Geometry: see drawing. Coordinates: mm, zero at the bounding-box minimum. A direction names the side the tool comes from. Round coordinates to 2 decimals unless told otherwise and drop trailing zeros. Loops run counter-clockwise (first coordinate to the right, second up) from the corner with the lowest first, then second, coordinate; pieces in that order, holes last.
(1) Set-up query: the marked faces 5 and 6. Return all of +Z, -Z, +X, -X, +Y, -Y with unobstructed straight access to the full face (end or side cutting, diameter ignored); none if empty.
(2) Section C-C, the plane x = 42.5. Return the cut outline in (y, z), plus the area to 3 significant figures.
(3) Material intervals for probe 1 along Y at (x, z) = (7.5, 13) (1 decimal); probe 2 along Y at (x, z) = (22, 44); probe 3 along X at (y, z) = (31.5, 40.5), sorted ascending.
(4) Section A-A, the plane z = 50.5. Return the cut outline in (x, y).
(5) Mould query, pull axis Y, two halves, no side actions, for the marked faces 1, 2, 3 and 4. Classes: pulls with the +Y half, pulls with the -Y half, needs draft (parallel to the pull), parting line crosses it, or undercut.
(6) Section B-B, the plane y = 40. Return the cut outline in (x, z), plus the area to 3 significant figures.
(7) Section D-D, the plane z = 32. Return the cut outline in (x, y).
(8) First-contact query: pin 1 Ø12 at (y, z) = (16.5, 15.5) entering from +X; pin 2 Ø6 at (y, z) = (41, 7.5) entering from -X; pin 3 Ø1.5 at (x, z) = (45, 35.5) entering from +Y. Flat tips, straight axial feed; report the tip coordinate or a pass-through.
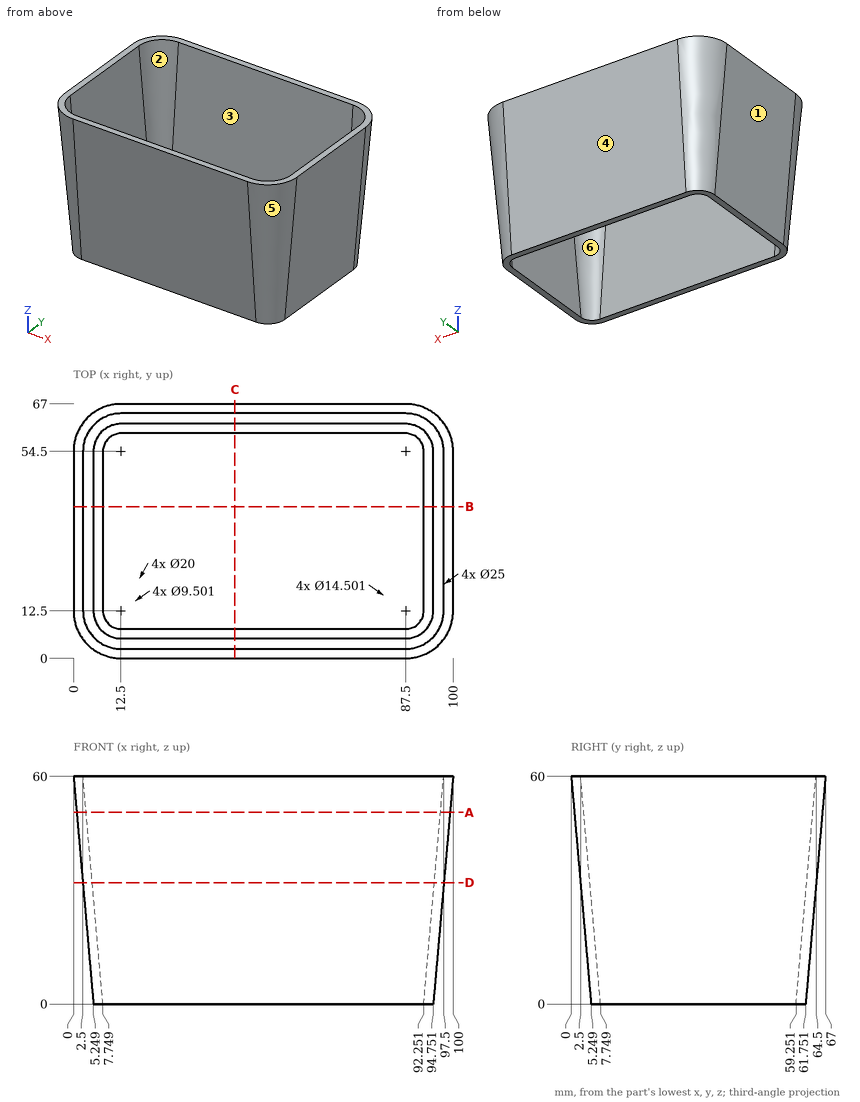
Output values:
1. face 5: -Z, +X, -Y
1. face 6: +Z
2. outline: (0, 60) - (5.25, 0) - (7.75, 0) - (2.5, 60) - close; (59.25, 0) - (61.75, 0) - (67, 60) - (64.5, 60) - close
2. area: 300 mm2
3. probe 1: y = 5.8 to 9.4, 57.6 to 61.2
3. probe 2: y = 1.4 to 3.9, 63.1 to 65.6
3. probe 3: x = 1.71 to 4.21, 95.79 to 98.29
4. outline: (0.83, 12.5) arc R11.67 ccw to (12.5, 0.83) - (87.5, 0.83) arc R11.67 ccw to (99.17, 12.5) - (99.17, 54.5) arc R11.67 ccw to (87.5, 66.17) - (12.5, 66.17) arc R11.67 ccw to (0.83, 54.5) - close; hole (3.33, 12.5) arc R9.17 ccw to (12.5, 3.33) - (87.5, 3.33) arc R9.17 ccw to (96.67, 12.5) - (96.67, 54.5) arc R9.17 ccw to (87.5, 63.67) - (12.5, 63.67) arc R9.17 ccw to (3.33, 54.5) - close
5. face 1: needs draft
5. face 2: undercut
5. face 3: undercut
5. face 4: pulls with the +Y half
6. outline: (0, 60) - (5.25, 0) - (7.75, 0) - (2.5, 60) - close; (92.25, 0) - (94.75, 0) - (100, 60) - (97.5, 60) - close
6. area: 300 mm2
7. outline: (2.45, 12.5) arc R10.05 ccw to (12.5, 2.45) - (87.5, 2.45) arc R10.05 ccw to (97.55, 12.5) - (97.55, 54.5) arc R10.05 ccw to (87.5, 64.55) - (12.5, 64.55) arc R10.05 ccw to (2.45, 54.5) - close; hole (4.95, 12.5) arc R7.55 ccw to (12.5, 4.95) - (87.5, 4.95) arc R7.55 ccw to (95.05, 12.5) - (95.05, 54.5) arc R7.55 ccw to (87.5, 62.05) - (12.5, 62.05) arc R7.55 ccw to (4.95, 54.5) - close
8. pin 1: stops at x = 96.63
8. pin 2: stops at x = 4.33
8. pin 3: stops at y = 64.92
